from build123d import *

# Parameters (mm, degrees)
F0_R      = 12.7
F11_DEPTH = 30.1625
F2_DEPTH  = 19.05
F4_DEPTH  = 41.275
F5_R      = 5.08
F6_R      = 7.874
F7_W      = 50.8
F7_H      = 22.3266
F8_DEPTH  = 38.1
F9_R      = 6.35
F10_DEPTH = 22.353


with BuildPart() as f11:
    # F0 (on Front) → F11 (new body, symmetric)
    with BuildSketch(Plane.XZ):
        with BuildLine():
            Line((85.852, 0), (22.352, 0))
            ThreePointArc((22.352, 0), (-15.805251, 15.805251), (0, -22.352))
            Line((0, -22.352), (91.8464, -22.352))
            Line((91.8464, -22.352), (85.852, 0))
        make_face()
        Circle(F0_R, mode=Mode.SUBTRACT)
        with BuildLine():
            ThreePointArc((131.0386, 34.798), (127.464415, 16.082358), (117.2464, 0))
            Line((117.2464, 0), (117.2464, -22.352))
            Line((117.2464, -22.352), (194.2084, -22.352))
            Line((194.2084, -22.352), (194.2084, 0))
            Line((194.2084, 0), (150.0886, 0))
            Line((150.0886, 0), (150.0886, 34.798))
            Line((150.0886, 34.798), (131.0386, 34.798))
        make_face()
        Polygon((117.2464, 0), (85.852, 0), (91.8464, -22.352), (117.2464, -22.352), align=None)
    extrude(amount=F11_DEPTH, both=True)

    # F1 (on face) → F2 (cut)
    with BuildSketch(Plane.XZ.offset(30.1625)):
        Polygon((117.2464, 0), (85.852, 0), (91.8464, -22.352), (117.2464, -22.352), align=None)
    extrude(amount=-F2_DEPTH, mode=Mode.SUBTRACT)

    # F3 (on face) → F4 (cut)
    with BuildSketch(Plane(origin=(0, 30.1625, 0), x_dir=(-1, 0, 0), z_dir=(0, 1, 0))):
        with BuildLine():
            Line((-150.0886, 34.798), (-150.0886, 0))
            Line((-150.0886, 0), (-117.2464, 0))
            ThreePointArc((-117.2464, 0), (-127.464415, 16.082358), (-131.0386, 34.798))
            Line((-131.0386, 34.798), (-150.0886, 34.798))
        make_face()
    extrude(amount=-F4_DEPTH, mode=Mode.SUBTRACT)

    # F5
    f5_edges = [f11.edges().sort_by_distance(p)[0] for p in [
        (22.352, 0, 0),
        (150.0886, -20.6375, 34.798),
        (150.0886, -20.6375, 0),
    ]]
    fillet(f5_edges, radius=F5_R)

    # F6
    f6_edges = [f11.edges().sort_by_distance(p)[0] for p in [
        (194.2084, 0, 0),
    ]]
    fillet(f6_edges, radius=F6_R)

    # F7 (on Top) → F8 (cut, symmetric)
    with BuildSketch(Plane.XY):
        with Locations((3.048, 0)):
            Rectangle(F7_W, F7_H)
    extrude(amount=F8_DEPTH, both=True, mode=Mode.SUBTRACT)

    # F9 (on face) → F10 (cut, through all)
    with BuildSketch(Plane.XY):
        with Locations((155.3464, 7.8105)):
            Circle(F9_R)
    extrude(amount=-F10_DEPTH, mode=Mode.SUBTRACT)


solid = f11.part
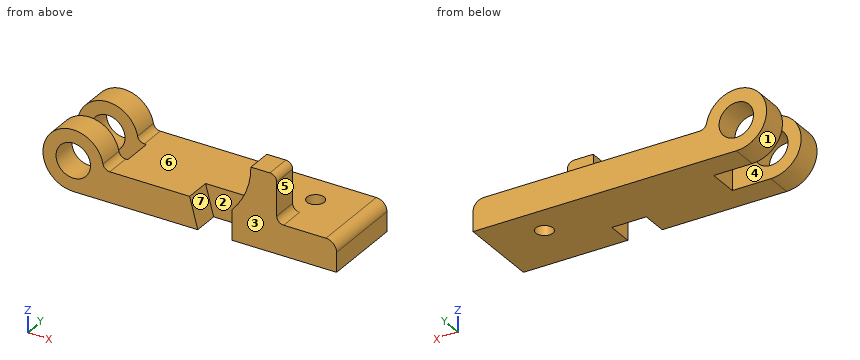
Can you work these out from the model? Positions are in its coordinate system, mm. Face numbers are marked on the shaded views. A direction names the side the tool comes from. Give positions to 0.01 mm unless a question says otherwise; leave off trailing zeros. Loops run counter-clockwise (first coordinate to the right, second up) from the corner with the lowest first, then second, coordinate; pieces in that order, holes last. Notation, with made-up numbers: (18.5, -33) - (32.5, -33) arc R32 ccw to (32.5, 2) - close; hole circle Ø1 at (76, 43.25). An arc over 180 degrees is marked (long way). Answer as a JSON object with one key per item and string values.
Q1. Imagine slicing it at D-D on z = -16.5. Write out the boundary of the cut face in (x, y), plus the area to 3 significant figures.
Geometry says:
{"outline": "(-15.08, -30.16) - (90.28, -30.16) - (90.28, -11.11) - (117.25, -11.11) - (117.25, -30.16) - (194.21, -30.16) - (194.21, 30.16) - (-15.08, 30.16) - (-15.08, 11.16) - (28.45, 11.16) - (28.45, -11.16) - (-15.08, -11.16) - close; hole circle Ø12.7 at (155.35, 7.81)", "area": "11,000 mm²"}
Q2. If I drill on L1, parallel to Z at x = 0, y = -19; L2, parallel to Y at x = 12, z = 17; L3, parallel to Z at x = 119, y = 14, over which ranges is the centre line in solid material (lowest first)?
Geometry says:
{"L1": "-22.35 to -12.7, 12.7 to 22.35", "L2": "-30.16 to -11.16, 11.16 to 30.16", "L3": "-22.35 to 0"}
Q3. Which directions (+Z, -Z, +X, -X, +Y, -Y) give clear straight access to the entire face, cutting with the end or side of a thin tool? Please do the marked faces 4, 5, 6 and 7.
Geometry says:
{"face 4": "+Z, -Z, -X", "face 5": "+Z, +X, +Y, -Y", "face 6": "+Z, +Y", "face 7": "+Z, -Y"}
Q4. Imagine slicing it at B-B on z = 10. Write out the boundary of the cut face in (x, y).
Geometry says:
{"outline": "(-19.99, -30.16) - (-7.83, -30.16) - (-7.83, -11.16) - (-19.99, -11.16) - close; (-19.99, 11.16) - (-7.83, 11.16) - (-7.83, 30.16) - (-19.99, 30.16) - close; (7.83, -30.16) - (19.99, -30.16) - (19.99, -11.16) - (7.83, -11.16) - close; (7.83, 11.16) - (19.99, 11.16) - (19.99, 30.16) - (7.83, 30.16) - close; (124.57, -30.16) - (150.09, -30.16) - (150.09, -11.11) - (124.57, -11.11) - close"}
Q5. If we mould it in two halves opening along X, with no side actions, what happens to the marked faces 1, 2 and 3? For each: pulls with the +X half, pulls with the -X half, needs draft (parallel to the pull), parting line crosses it, or undercut.
Geometry says:
{"face 1": "parting line crosses it", "face 2": "undercut", "face 3": "needs draft"}
Q6. Imagine slicing it at C-C on y = 17. Write out the boundary of the cut face in (x, z), plus the area to 3 significant figures.
Geometry says:
{"outline": "(0, -22.35) - (194.21, -22.35) - (194.21, -7.87) arc R7.87 ccw to (186.33, 0) - (26.96, 0) arc R5.08 cw to (21.97, 4.14) arc R22.35 ccw (long way) to start; hole circle Ø25.4 at (0, 0)", "area": "5,000 mm²"}
Q7. Imagine slicing it at A-A on y = -14. Write out the boundary of the cut face in (x, z).
Geometry says:
{"outline": "(0, -22.35) - (91.85, -22.35) - (85.85, 0) - (26.96, 0) arc R5.08 cw to (21.97, 4.14) arc R22.35 ccw (long way) to start; (117.25, -22.35) - (194.21, -22.35) - (194.21, -7.87) arc R7.87 ccw to (186.33, 0) - (155.17, 0) arc R5.08 cw to (150.09, 5.08) - (150.09, 29.72) arc R5.08 ccw to (145.01, 34.8) - (131.04, 34.8) arc R50.8 cw to (117.25, 0) - close; hole circle Ø25.4 at (0, 0)"}
Q8. Will these pins go through, and if not, where does the flat tip stop? P1, Ø18, axis at y = 4.5, z = -11.5, coming from the -X side; P2, Ø12, axis at x = 31.5, z = 7, coming from the +Y side; P3, Ø15, axis at y = -24.5, z = 12, coming from the +X side; P4, Ø9.5, axis at y = -25, z = -11, coming from the -X side.
Geometry says:
{"P1": "x = -21.68", "P2": "through", "P3": "x = 150.12", "P4": "x = -21.46"}
